```python
from build123d import *


with BuildPart() as part:
    # Sketch1 → Revolve1 (revolve)
    with BuildSketch(Plane.XY, mode=Mode.PRIVATE) as revolve1_sk:
        Polygon((-94.064695228, 790), (0, 790), (0, 800), (-100, 800), (-185, 32.501032947), (-185, -27.498967053), (-178, -27.498967053), (-178, 32.501032947), (-171.350171875, 92.501032947), (-20, 92.501032947), (-20, 570), (-118.429548867, 570), align=None)
        Polygon((-119.537042214, 560), (-27, 560), (-27, 102.501032947), (-170.241867187, 102.501032947), align=None, mode=Mode.SUBTRACT)
    revolve(revolve1_sk.sketch.rotate(Axis((0, -27.498967053, 0), (0, 1, 0)), 270), axis=Axis((0, -27.498967053, 0), (0, 1, 0)))


solid = part.part
```
Build history of the part. All positions in model axes, mm. A direction names the side the tool comes from. Give positions to 0.01 mm unless a question says otherwise; leave off trailing zeros. Loops run counter-clockwise (first coordinate to the right, second up) from the corner with the lowest first, then second, coordinate; pieces in that order, holes last.
1) Two-plate mould, pull along Y, no slides. Class faces 1 (the face through (19.524, 334.593, 4.336)), 2 (the face through (-1, 800, -1)), 3 (the face through (-28, 560, 2)): released by +Y, released by -Y, zero draft, split by the parting line, or undercut.
Values follow:
face 1: zero draft
face 2: released by +Y
face 3: undercut
2) Band-saw the part on C-C on x = 44. State how many separate pieces and enclosed holes the cut face has, then the cut area to 3 significant figures.
Values follow:
separate pieces: 1
enclosed holes: 2
area: 19,500 mm2
3) Drop flat-ended pins along their axis: P1, Ø3, axis at x = 53, y = 122, coming from the +Z side; P2, Ø2, axis at x = -59.5, z = -81, coming from the -Y side; P3, Ø5, axis at y = 82, z = -62.5, coming from the +X side. Give the stop position or say it passes through.
Values follow:
P1: stops at z = 167.37
P2: stops at y = 92.5
P3: stops at x = 169.24
4) Probe line 1 along Y through (x, z) = (18.5, -54.5); line 2 along X through (y, z) = (-6, 0); line 3 along X through (y, z) = (336, -10). List the from-to ranges inside material, lowest first.
Values follow:
line 1: y = 92.5 to 102.5, 560 to 570, 790 to 800
line 2: x = -185 to -178, 178 to 185
line 3: x = -151.06 to -144.02, -25.08 to -17.32, 17.32 to 25.08, 144.02 to 151.06
5) Band-saw the part on B-B on x = 0. List the corners of the cut face in (y, z).
Values follow:
outline: (-27.5, -185) - (32.5, -185) - (800, -100) - (800, 100) - (32.5, 185) - (-27.5, 185) - (-27.5, 178) - (32.5, 178) - (92.5, 171.35) - (92.5, 20) - (570, 20) - (570, 118.43) - (790, 94.06) - (790, -94.06) - (570, -118.43) - (570, -20) - (92.5, -20) - (92.5, -171.35) - (32.5, -178) - (-27.5, -178) - close; hole (102.5, -170.24) - (560, -119.54) - (560, -27) - (102.5, -27) - close; hole (102.5, 27) - (560, 27) - (560, 119.54) - (102.5, 170.24) - close
6) 3-axis set-ups, long thin cutter, end or side, ignore diameter. For faces 4 (the face through (26.36, 328.05, 5.85)), 5 (the face through (-120.301, 2.921, 131.193)), 6 (the face through (180.6, 2.1, 40.1)): which of +Z, -Z, +X, -X, +Y, -Y reach the whole face in a straight line?
Values follow:
face 4: none
face 5: -Y
face 6: +Y, -Y
7) Band-saw the part on A-A on z = 0. List the corners of the cut face in (x, y), then the cut area to 3 significant figures.
Values follow:
outline: (-185, -27.5) - (-178, -27.5) - (-178, 32.5) - (-171.35, 92.5) - (-20, 92.5) - (-20, 570) - (-118.43, 570) - (-94.06, 790) - (94.06, 790) - (118.43, 570) - (20, 570) - (20, 92.5) - (171.35, 92.5) - (178, 32.5) - (178, -27.5) - (185, -27.5) - (185, 32.5) - (100, 800) - (-100, 800) - (-185, 32.5) - close; hole (-170.24, 102.5) - (-27, 102.5) - (-27, 560) - (-119.54, 560) - close; hole (27, 102.5) - (170.24, 102.5) - (119.54, 560) - (27, 560) - close
area: 24,900 mm2
